Print and shaded views of the part. All mm, measured from the part's lowest x, y and z. Coordinates: 2 decimals unless noted, no trailing zeros. Order: outer loops, then holes, each group sorted by start corner. A loop starts at its lowest first (then second) coordinate and runs counter-clockwise, first axis right, second up. Notation, with made-up numbers: M -9,-38 L 47,-38 A16 cw 47,-13 Z; hole C 32,22.5 d7. An arc over 180 degrees is marked long. Use a Markdown table: item, result. Add a question column.
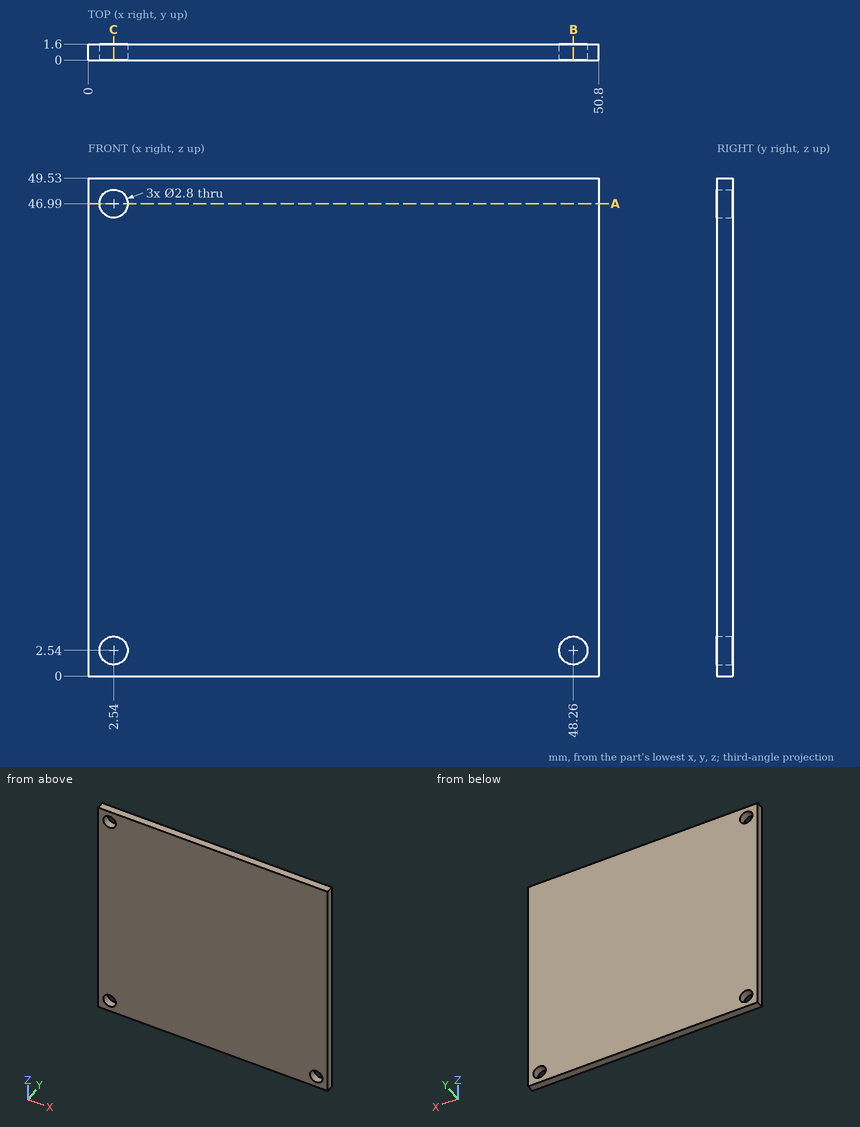
(1) Drill centre lines: line 1 along Z through (x, y) = (2.54, 0.7); line 2 along X through (y, z) = (1.25, 2.54); line 3 along Z through (x, y) = (48.26, 0.9). Where is each one in solid material? Low to high. Write a range as from..to.
(2) Drop a flat-ended pin along its axis: P1, Ø2, axis at x = 2.54, z = 46.99, coming from the +Y side. Give the stop position or say it passes through.
(3) Slice it at C-C on x = 2.54. Give the cut face in (y, z), and give its area (3 significant figures).
(4) Slice it at A-A on z = 46.99. Give the cut face in (x, y), and give its area (3 significant figures).
(5) Slice it at B-B on x = 48.26. Give the cut face in (y, z).
Solutions:
| question | item | result |
|---|---|---|
| 1 | line 1 | 0..1.14, 3.94..45.59, 48.39..49.53 |
| 1 | line 2 | 0..1.14, 3.94..46.86, 49.66..50.8 |
| 1 | line 3 | 0..1.14, 3.94..49.53 |
| 2 | P1 | through |
| 3 | outline | M 0,0 L 1.6,0 L 1.6,1.14 L 0,1.14 Z; M 0,3.94 L 1.6,3.94 L 1.6,45.59 L 0,45.59 Z; M 0,48.39 L 1.6,48.39 L 1.6,49.53 L 0,49.53 Z |
| 3 | area | 70.3 mm² |
| 4 | outline | M 0,0 L 1.14,0 L 1.14,1.6 L 0,1.6 Z; M 3.94,0 L 50.8,0 L 50.8,1.6 L 3.94,1.6 Z |
| 4 | area | 76.8 mm² |
| 5 | outline | M 0,0 L 1.6,0 L 1.6,1.14 L 0,1.14 Z; M 0,3.94 L 1.6,3.94 L 1.6,49.53 L 0,49.53 Z |
